from build123d import *

# Parameters (mm, degrees)
EXTRUDE_THIN1_DEPTH = 46
SKETCH2_R           = 1
CUT_EXTRUDE1_DEPTH  = 49.523190332
SKETCH3_R           = 1.5
CUT_EXTRUDE2_DEPTH  = 49.961719741
CUT_EXTRUDE3_DEPTH  = 49.961719741


with BuildPart() as part:
    # Sketch1 → Extrude-Thin1 (new body)
    with BuildSketch(Plane.XY):
        Polygon((0, 15), (0, 0), (7.5, 0), (7.5, 1.5), (1.5, 1.5), (1.5, 15), align=None)
    extrude(amount=EXTRUDE_THIN1_DEPTH)

    # Sketch2 → Cut-Extrude1 (cut, through all)
    with BuildSketch(Plane(origin=(0, 1.5, 0), x_dir=(1, 0, 0), z_dir=(0, 1, 0))):
        with Locations(Location((3.75, -9, 0), (0, 0, 270))):
            Circle(SKETCH2_R)
        with Locations(Location((3.75, -37, 0), (0, 0, 90))):
            Circle(SKETCH2_R)
    extrude(amount=-CUT_EXTRUDE1_DEPTH, mode=Mode.SUBTRACT)

    # Sketch3 → Cut-Extrude2 (cut, through all)
    with BuildSketch(Plane.ZY):
        with Locations((41.5, 8.25)):
            Circle(SKETCH3_R)
        with Locations((4.5, 8.25)):
            Circle(SKETCH3_R)
    extrude(amount=-CUT_EXTRUDE2_DEPTH, mode=Mode.SUBTRACT)

    # Sketch4 → Cut-Extrude3 (cut, through all)
    with BuildSketch(Plane.ZY):
        Polygon((0, 12), (3, 15), (0, 15), align=None)
        Polygon((46, 15), (43, 15), (46, 12), align=None)
    extrude(amount=-CUT_EXTRUDE3_DEPTH, mode=Mode.SUBTRACT)


solid = part.part
Input: part model. Units: mm. Frame: model coordinates. A direction names the side the tool comes from. Give positions to 0.01 mm unless a question says otherwise; leave off trailing zeros. Order: outer loops, then holes, each group sorted by start corner. A loop starts at its lowest first (then second) coordinate and runs counter-clockwise, first axis right, second up. Notation, with made-up numbers: (-2, 64.5) -> (49, 64.5) arc R20 ccw to (49, 86.5) -> close; hole circle Ø7 at (-8, -31.75). An arc over 180 degrees is marked (long way). Use one line per item in the form item = value.
1) Section A-A, the plane z = 9. Return loops of the section in (x, y), and give its area (3 significant figures).
Response values:
outline = (0, 0) -> (2.75, 0) -> (2.75, 1.5) -> (1.5, 1.5) -> (1.5, 15) -> (0, 15) -> close; (4.75, 0) -> (7.5, 0) -> (7.5, 1.5) -> (4.75, 1.5) -> close
area = 28.5 mm^2
2) Reachability of faces 4 (the flat face through (1.5, 8, 23)), 5 (the cylindrical face through (0.74, 7.34, 40.31)) from +Z, -Z, +X, -X, +Y, -Y: full face, straight path, thin tool, end or side. Return the list, or none.
Response values:
face_4 = +Z, -Z, +X, +Y
face_5 = +X, -X
3) Mould query, pull axis Z, two halves, no side actions, for faces 1 (the flat face through (4, 0, 23)), 2 (the flat face through (1, 5, 46)), 3 (the cylindrical face through (3.45, 0.76, 36.046)). Classes: pulls with the +Z half, pulls with the -Z half, needs draft (parallel to the pull), parting line crosses it, or undercut.
Response values:
face_1 = needs draft
face_2 = pulls with the +Z half
face_3 = undercut
4) Line query: probe 1 along X at (y, z) = (0.5, 9); probe 2 along Y at (x, z) = (0.65, 4.5); probe 3 along X at (y, z) = (4.75, 6.5). Output: solid intervals per line, ascending.
Response values:
probe_1 = 0 to 2.75, 4.75 to 7.5
probe_2 = 0 to 6.75, 9.75 to 15
probe_3 = 0 to 1.5
5) Section D-D, the plane y = 1. Return loops of the section in (x, z).
Response values:
outline = (0, 0) -> (7.5, 0) -> (7.5, 46) -> (0, 46) -> close; hole circle Ø2 at (3.75, 9); hole circle Ø2 at (3.75, 37)
6) Section C-C, the plane x = 3.75. Return loops of the section in (y, z).
Response values:
outline = (0, 0) -> (1.5, 0) -> (1.5, 8) -> (0, 8) -> close; (0, 10) -> (1.5, 10) -> (1.5, 36) -> (0, 36) -> close; (0, 38) -> (1.5, 38) -> (1.5, 46) -> (0, 46) -> close
7) First-contact query: pin 1 Ø2.5 at (x, z) = (3.75, 37) entering from +Y; pin 2 Ø1.6 at (x, z) = (3.75, 9) entering from -Y; pin 3 Ø5 at (y, z) = (8.25, 41.5) entering from +X. Flat tips, straight axial feed; report the tip coordinate or a pass-through.
Response values:
pin_1 = 1.5
pin_2 = through
pin_3 = 1.5
8) Section B-B, the plane y = 8.25. Return loops of the section in (x, z), and give its area (3 significant figures).
Response values:
outline = (0, 0) -> (1.5, 0) -> (1.5, 3) -> (0, 3) -> close; (0, 6) -> (1.5, 6) -> (1.5, 40) -> (0, 40) -> close; (0, 43) -> (1.5, 43) -> (1.5, 46) -> (0, 46) -> close
area = 60.0 mm^2
